from build123d import *

# Parameters (mm, degrees)
SKETCH2_W           = 230
SKETCH2_H           = 230
BOSS_EXTRUDE1_DEPTH = 5
SKETCH3_R           = 3
CUT_EXTRUDE1_DEPTH  = 326.307546792
SKETCH4_R           = 3
CUT_EXTRUDE2_DEPTH  = 326.307546792
SKETCH5_R           = 3
CUT_EXTRUDE3_DEPTH  = 326.307546792
SKETCH6_R           = 3
CUT_EXTRUDE4_DEPTH  = 326.307546792


with BuildPart() as part:
    # Sketch2 → Boss-Extrude1 (new body)
    with BuildSketch(Plane(origin=(0, 0, 0), x_dir=(1, 0, 0), z_dir=(0, 1, 0))):
        with Locations((115, 115)):
            Rectangle(SKETCH2_W, SKETCH2_H)
    extrude(amount=BOSS_EXTRUDE1_DEPTH)

    # Sketch3 → Cut-Extrude1 (cut, through all)
    with BuildSketch(Plane(origin=(0, 5, 0), x_dir=(1, 0, 0), z_dir=(0, 1, 0))):
        with Locations(Location((6, 224, 0), (0, 0, 270))):
            Circle(SKETCH3_R)
    extrude(amount=-CUT_EXTRUDE1_DEPTH, mode=Mode.SUBTRACT)

    # Sketch4 → Cut-Extrude2 (cut, through all)
    with BuildSketch(Plane(origin=(0, 5, 0), x_dir=(1, 0, 0), z_dir=(0, 1, 0))):
        with Locations(Location((224, 224, 0), (0, 0, 270))):
            Circle(SKETCH4_R)
    extrude(amount=-CUT_EXTRUDE2_DEPTH, mode=Mode.SUBTRACT)

    # Sketch5 → Cut-Extrude3 (cut, through all)
    with BuildSketch(Plane(origin=(0, 5, 0), x_dir=(1, 0, 0), z_dir=(0, 1, 0))):
        with Locations(Location((6, 6, 0), (0, 0, 270))):
            Circle(SKETCH5_R)
    extrude(amount=-CUT_EXTRUDE3_DEPTH, mode=Mode.SUBTRACT)

    # Sketch6 → Cut-Extrude4 (cut, through all)
    with BuildSketch(Plane(origin=(0, 5, 0), x_dir=(1, 0, 0), z_dir=(0, 1, 0))):
        with Locations(Location((224, 6, 0), (0, 0, 270))):
            Circle(SKETCH6_R)
    extrude(amount=-CUT_EXTRUDE4_DEPTH, mode=Mode.SUBTRACT)


solid = part.part
Work out the finished part from the listing and answer in its coordinate system (mm). Round coordinates to 2 decimals unless told otherwise and drop trailing zeros. Write each loop counter-clockwise with the first axis right and the second up, starting at its lowest first coordinate (ties: lowest second). Pieces come first, ordered by that corner, then holes. Notation, with made-up numbers: M 40.25,14 L 70.25,14 A32 cw 70.25,43 Z; hole C -8,21.5 d10. An arc over 180 degrees is marked long. Use a Markdown table: item, result.
1) The part is cut by section B-B on z = -6. Give the vertices of the cut face in (x, y), plus the area to 3 significant figures.
Taken from the geometry:
| item | result |
|---|---|
| outline | M 0,0 L 3,0 L 3,5 L 0,5 Z; M 9,0 L 221,0 L 221,5 L 9,5 Z; M 227,0 L 230,0 L 230,5 L 227,5 Z |
| area | 1,090 mm2 |
2) Consider line 1 (Z direction, x = 224, y = 2.9); line 2 (X direction, y = 3.35, z = -224). Determine where each line is inside the solid, lowest interval first. Write a range as [from, to].
Taken from the geometry:
| item | result |
|---|---|
| line 1 | z = [-230, -227], [-221, -9], [-3, 0] |
| line 2 | x = [0, 3], [9, 221], [227, 230] |
3) Determine the mould class of faces 1 (the face through (0, 2, -113)), 2 (the face through (3.338, 2.535, -4.616)), 3 (the face through (230, 2, -113)) for opening direction X: pulls with the +X half, pulls with the -X half, needs draft (parallel to the pull), parting line crosses it, or undercut.
Taken from the geometry:
| item | result |
|---|---|
| face 1 | pulls with the -X half |
| face 2 | undercut |
| face 3 | pulls with the +X half |
4) A flat-ended cylindrical pin translates along its axis: pin 1 (12 mm diameter, centred on x = 136.5, z = -171.5, fed in from -Y). Find the tip coordinate at first contact, or state that the pin passes through.
Taken from the geometry:
| item | result |
|---|---|
| pin 1 | stops at y = 0 |
5) The part is cut by section A-A on x = 6. Give the vertices of the cut face in (y, z).
Taken from the geometry:
| item | result |
|---|---|
| outline | M 0,-230 L 5,-230 L 5,-227 L 0,-227 Z; M 0,-221 L 5,-221 L 5,-9 L 0,-9 Z; M 0,-3 L 5,-3 L 5,0 L 0,0 Z |
